Could you check a few things on this model? Use its own coordinates, in mm. Face numbers are marked on the shaded views. A direction names the side the tool comes from. Give positions to 0.01 mm unless a question says otherwise; leave off trailing zeros. Write each loop counter-clockwise with the first axis right and the second up, starting at its lowest first coordinate (ties: lowest second). Pieces come first, ordered by that corner, then holes. Notation, with made-up numbers: (-8, 51) - (25, 51) arc R7 ccw to (25, 61) - close; hole circle Ø6 at (73.25, 33). An arc over 180 degrees is marked (long way). Write item = value, one per line.
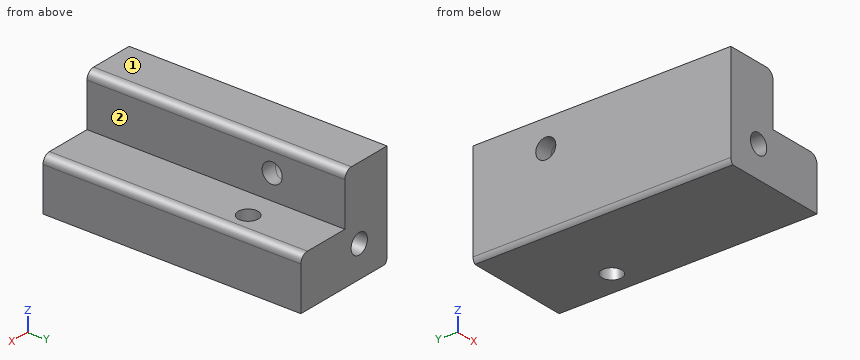
from build123d import *

# Parameters (mm, degrees)
HOLE_TOPMAIN_OUTLINE_W = 12.9
HOLE_TOPMAIN_OUTLINE_H = 12.9
HOLE_TOPMAIN_OUTLINE_R = 2.5
HOLE_TOPMAIN_DEPTH     = 64.27
SKETCH14_R             = 2.5
CUT_EXTRUDE9_DEPTH     = 67.100627077
SKETCH15_R             = 3.25
CUT_EXTRUDE10_DEPTH    = 66.309210028
SKETCH18_W             = 12.9
SKETCH18_H             = 64.27
SKETCH18_R             = 3.25
BOSS_EXTRUDE2_DEPTH    = 13.5
FILLET3_R              = 2
SKETCH19_R             = 2.5
CUT_EXTRUDE11_DEPTH    = 13.5
SKETCH22_W             = 13.5
SKETCH22_H             = 64.27
BOSS_EXTRUDE3_DEPTH    = 13.5
BOSS_EXTRUDE5_START    = -26.4
SKETCH24_R             = 3.25
BOSS_EXTRUDE5_DEPTH    = 26.4
CUT_EXTRUDE12_START    = -64.27
SKETCH25_R             = 2.5
CUT_EXTRUDE12_DEPTH    = 64.27
SKETCH26_R             = 2.5
CUT_EXTRUDE13_DEPTH    = 13.5
SKETCH28_R             = 2.5
CUT_EXTRUDE14_DEPTH    = 13.5
FILLET4_R              = 2
SKETCH31_W             = 26.4
SKETCH31_H             = 0.6
CUT_EXTRUDE15_DEPTH    = 64.27


# Read off the part's stored shape, not the designer's step: hole-TopMain
with BuildPart() as part:
    # hole-TopMain outline → hole-TopMain (new body)
    with BuildSketch(Plane(origin=(0, 0, 0), x_dir=(1, 0, 0), z_dir=(0, 1, 0))):
        with Locations((-2.05, 2.05)):
            Rectangle(HOLE_TOPMAIN_OUTLINE_W, HOLE_TOPMAIN_OUTLINE_H)
        Circle(HOLE_TOPMAIN_OUTLINE_R, mode=Mode.SUBTRACT)
    extrude(amount=HOLE_TOPMAIN_DEPTH)

    # Sketch14 → Cut-Extrude9 (cut, through all)
    with BuildSketch(Plane(origin=(0, 0, -8.5), x_dir=(-1, 0, 0), z_dir=(0, 0, -1))):
        with Locations((1.75, 46.135)):
            Circle(SKETCH14_R)
    extrude(amount=-CUT_EXTRUDE9_DEPTH, mode=Mode.SUBTRACT)

    # Sketch15 → Cut-Extrude10 (cut, through all)
    with BuildSketch(Plane(origin=(0, 0, -3.5), x_dir=(-1, 0, 0), z_dir=(0, 0, -1))):
        with Locations((1.75, 46.135)):
            Circle(SKETCH15_R)
    extrude(amount=-CUT_EXTRUDE10_DEPTH, mode=Mode.SUBTRACT)

    # Sketch18 → Boss-Extrude2 (add)
    with BuildSketch(Plane.XY.offset(4.4)):
        with Locations((-2.05, 32.135)):
            Rectangle(SKETCH18_W, SKETCH18_H)
        with Locations(Location((-1.75, 46.135, 0), (0, 0, 180))):
            Circle(SKETCH18_R, mode=Mode.SUBTRACT)
    extrude(amount=BOSS_EXTRUDE2_DEPTH)

    # Fillet3
    fillet3_edges = [part.edges().sort_by_distance(p)[0] for p in [
        (-8.5, 32.135, -8.5),
        (4.4, 32.135, 17.9),
    ]]
    fillet(fillet3_edges, radius=FILLET3_R)

    # Sketch19 → Cut-Extrude11 (cut)
    with BuildSketch(Plane.ZY.offset(8.5)):
        with Locations((11.15, 46.135)):
            Circle(SKETCH19_R)
    extrude(amount=-CUT_EXTRUDE11_DEPTH, mode=Mode.SUBTRACT)

    # Sketch22 → Boss-Extrude3 (add)
    with BuildSketch(Plane(origin=(4.4, 0, 0), x_dir=(0, 0, -1), z_dir=(1, 0, 0))):
        with Locations((1.75, 32.135)):
            Rectangle(SKETCH22_W, SKETCH22_H)
    extrude(amount=BOSS_EXTRUDE3_DEPTH)

    # Sketch24 → Boss-Extrude5 (add)
    with BuildSketch(Plane.XY.offset(17.9).offset(BOSS_EXTRUDE5_START)):
        with Locations((-1.75, 46.135)):
            Circle(SKETCH24_R)
    extrude(amount=BOSS_EXTRUDE5_DEPTH)

    # Sketch25 → Cut-Extrude12 (cut)
    with BuildSketch(Plane(origin=(0, 64.27, 0), x_dir=(1, 0, 0), z_dir=(0, 1, 0)).offset(CUT_EXTRUDE12_START)):
        with Locations(Location((0, 0, 0), (0, 0, 90))):
            Circle(SKETCH25_R)
    extrude(amount=CUT_EXTRUDE12_DEPTH, mode=Mode.SUBTRACT)

    # Sketch26 → Cut-Extrude13 (cut)
    with BuildSketch(Plane.ZY.offset(8.5)):
        with Locations((11.15, 46.135)):
            Circle(SKETCH26_R)
    extrude(amount=-CUT_EXTRUDE13_DEPTH, mode=Mode.SUBTRACT)

    # Sketch28 → Cut-Extrude14 (cut)
    with BuildSketch(Plane(origin=(0, 0, -8.5), x_dir=(-1, 0, 0), z_dir=(0, 0, -1))):
        with Locations((-11.75, 46.135)):
            Circle(SKETCH28_R)
    extrude(amount=-CUT_EXTRUDE14_DEPTH, mode=Mode.SUBTRACT)

    # Fillet4
    fillet4_edges = [part.edges().sort_by_distance(p)[0] for p in [
        (17.9, 32.135, 5),
    ]]
    fillet(fillet4_edges, radius=FILLET4_R)

    # Sketch31 → Cut-Extrude15 (cut)
    with BuildSketch(Plane(origin=(0, 64.27, 0), x_dir=(1, 0, 0), z_dir=(0, 1, 0))):
        with Locations((4.7, 8.2)):
            Rectangle(SKETCH31_W, SKETCH31_H)
    extrude(amount=-CUT_EXTRUDE15_DEPTH, mode=Mode.SUBTRACT)


solid = part.part
1. For pin 1 (3 mm diameter, centred on y = 46.135, z = 11.15, fed in from +X); pin 2 (6 mm diameter, centred on x = 3, y = 31.5, fed in from +Z); pin 3 (1 mm diameter, centred on x = 7, y = 18.5, fed in from +Z); pin 4 (3.5 mm diameter, centred on y = 47, z = 11.5, fed in from +X), each with a flat end and sliding along its axis, tell me the tip position at first contact or that it passes through.
Filled sheet:
pin_1 = through
pin_2 = 17.9
pin_3 = 5
pin_4 = 4.4
2. If we section it at A-A, the plane y = 47.5: Please give me the cut outline in (x, z), and give its area (3 significant figures).
Filled sheet:
outline = (-8.5, -6.5) arc R2 ccw to (-7.93, -7.9) - (9.66, -7.9) - (9.66, 5) - (4.4, 5) - (4.4, 9.06) - (-8.5, 9.06) - close; (-8.5, 13.24) - (4.4, 13.24) - (4.4, 15.9) arc R2 ccw to (2.4, 17.9) - (-8.5, 17.9) - close; (13.84, -7.9) - (17.9, -7.9) - (17.9, 3) arc R2 ccw to (15.9, 5) - (13.84, 5) - close; hole circle Ø5 at (0, 0)
area = 377 mm2
3. If we section it at B-B, the plane z = 0: Please give me the cut outline in (x, y) (3 decimals), and give its area (3 significant figures).
Filled sheet:
outline = (-8.5, 0) - (-2.5, 0) - (-2.5, 64.27) - (-8.5, 64.27) - close; (2.5, 0) - (17.9, 0) - (17.9, 64.27) - (2.5, 64.27) - close; hole circle Ø5 at (11.75, 46.135)
area = 1,360 mm2
4. I need wall thicknesses on line 1 (Y direction, x = -0.5, z = 11.15) (3 decimals); line 2 (X direction, y = 59, z = 16); line 3 (Z direction, x = 15.25, y = 29). Which ranges of each line are inside material? Lowest first, please.
Filled sheet:
line_1 = 0 to 43.635, 48.635 to 64.27
line_2 = -8.5 to 4.4
line_3 = -7.9 to 5
5. Which directions (+Z, -Z, +X, -X, +Y, -Y) give clear straight access to the entire face, cutting with the end or side of a thin tool? Please do the marked faces 1 and 2.
Filled sheet:
face_1 = +Z, +X, -X, +Y, -Y
face_2 = +Z, +X, +Y, -Y
6. If we section it at C-C, the plane x = 11.75: Please give me the cut outline in (y, z) (3 decimals).
Filled sheet:
outline = (0, -7.9) - (43.635, -7.9) - (43.635, 5) - (0, 5) - close; (48.635, -7.9) - (64.27, -7.9) - (64.27, 5) - (48.635, 5) - close
7. If we section it at D-D, the plane z = 11.15: Please give me the cut outline in (x, y) (3 decimals).
Filled sheet:
outline = (-8.5, 0) - (4.4, 0) - (4.4, 43.635) - (-8.5, 43.635) - close; (-8.5, 48.635) - (4.4, 48.635) - (4.4, 64.27) - (-8.5, 64.27) - close
